Autodesk Inventor part; units mm, degrees
ref_plane "YZ Plane" through (0, 0, 0) normal (1, 0, 0) x (0, 1, 0)
ref_plane "XZ Plane" through (0, 0, 0) normal (0, 1, 0) x (-1, 0, 0)
ref_plane "XY Plane" through (0, 0, 0) normal (0, 0, 1) x (1, 0, 0)
sketch "Sketch1" plane through (0, 0, 0) normal (1, 0, 0) x (0, 1, 0)
  circle A0 centre (-31.75, 44.45) radius 11.1125
  circle A1 centre (-76.2, 44.45) radius 11.1125
  circle A2 centre (-101.6, 44.45) radius 11.1125
  line L0 (-130.175, 71.4375) -> (-92.075, 71.4375)
  arc A3 (-130.175, 71.4375) -> (-134.9375, 66.675) centre (-130.175, 66.675) ccw
  arc A4 (26.9875, 17.4625) -> (31.75, 22.225) centre (26.9875, 22.225) ccw
  line L1 (-130.175, 17.4625) -> (-92.075, 17.4625)
  circle A5 centre (25.4, 28.575) radius 2.1082
  circle A6 centre (-92.075, 66.675) radius 2.1082
  line L2 (31.75, 66.675) -> (31.75, 22.225)
  circle A7 centre (-92.075, 22.225) radius 2.1082
  arc A8 (-134.9375, 22.225) -> (-130.175, 17.4625) centre (-130.175, 22.225) ccw
  circle A9 centre (-130.175, 66.675) radius 2.1082
  line L3 (-134.9375, 66.675) -> (-134.9375, 22.225)
  circle A10 centre (-130.175, 22.225) radius 2.1082
  line L4 (-92.075, 71.4375) -> (26.9875, 71.4375)
  arc A11 (31.75, 66.675) -> (26.9875, 71.4375) centre (26.9875, 66.675) ccw
  circle A12 centre (26.9875, 66.675) radius 2.1345
  line L5 (-92.075, 17.4625) -> (26.9875, 17.4625)
  line L6 (26.9875, 66.675) -> (-17.4625, 66.675)
  line L7 (-17.4625, 66.675) -> (-11.1125, 66.675)
  line L8 (-17.4625, 66.675) -> (-23.8125, 66.675)
  circle A13 centre (-11.1125, 66.675) radius 2.1345
  line L9 (26.9875, 44.45) -> (6.6675, 44.45)
  circle A14 centre (6.6675, 44.45) radius 14.2875
  line L10 (-130.175, 22.225) -> (-92.075, 22.225)
  line L11 (-111.125, 22.225) -> (-111.125, 6.35)
  circle A15 centre (-111.125, 6.35) radius 2.1336
  line L12 (-111.125, 6.35) -> (-111.125, 0)
  line L13 (-111.125, 0) -> (-117.475, 0)
  line L14 (-111.125, 0) -> (-104.775, 0)
  line L15 (-117.475, 0) -> (-130.175, 17.4625)
  line L16 (-104.775, 0) -> (-92.075, 17.4625)
  line L17 (-130.175, 66.675) -> (-92.075, 66.675)
  line L18 (-111.125, 66.675) -> (-111.125, 82.55)
  circle A16 centre (-111.125, 82.55) radius 2.1336
  line L19 (-111.125, 82.55) -> (-111.125, 88.9)
  line L20 (-111.125, 88.9) -> (-117.475, 88.9)
  line L21 (-117.475, 88.9) -> (-104.775, 88.9)
  line L22 (-104.775, 88.9) -> (-92.075, 71.4375)
  line L23 (-117.475, 88.9) -> (-130.175, 71.4375)
  line L24 (26.9875, 71.4375) -> (55.5625, 71.4375)
  line L25 (55.5625, 71.4375) -> (55.5625, 58.7375)
  line L26 (55.5625, 58.7375) -> (31.75, 58.7375)
  line L27 (55.5625, 65.0875) -> (49.2125, 65.0875)
  circle A17 centre (49.2125, 65.0875) radius 2.1336
  point P0 (0, 0)
  point P1 (26.9875, 71.4375)
  dimension "d2" = 6.35
  dimension "d3" = 6.35
  dimension "d4" = 44.45
  dimension "d5" = 20.32
  dimension "d6" = 28.575
  dimension "d7" = 4.2672
  dimension "d8" = 6.35
  dimension "d9" = 6.35
  dimension "d10" = 6.35
  dimension "d11" = 15.875
  dimension "d12" = 4.2672
  dimension "d13" = 6.35
  dimension "d14" = 6.35
  dimension "d15" = 12.7
  dimension "d21" = 28.575
  dimension "d22" = 6.35
  dimension "d23" = 4.2672
extrude "Extrusion1" add sketch "Sketch1" along normal blind 3.175 contours L23 L20 L19 A16 L18 L0 | L0 L4 A11 L2 A4 L5 L1 A8 L3 A3 | L18 A16 L19 L21 L22 L0 | L24 L25 L26 L2 A11
fillet "Fillet1" radius 6.35 4 edges at (1.5875, -130.175, 71.4375) (1.5875, -117.475, 88.9) (1.5875, -104.775, 88.9) (1.5875, -92.075, 71.4375)
fillet "Fillet3" radius 6.35 3 edges at (1.5875, 31.75, 58.7375) (1.5875, 55.5625, 58.7375) (1.5875, 55.5625, 71.4375)
properties part number "winch plate"
Model file for the job. Use its own axes, mm. A direction names the side the tool comes from. Give positions to 0.01 mm unless a question says otherwise; leave off trailing zeros. Order: outer loops, then holes, each group sorted by start corner. A loop starts at its lowest first (then second) coordinate and runs counter-clockwise, first axis right, second up. Notation, with made-up numbers: (37.5, 86) -> (63.5, 86) arc R25 cw to (63.5, 118) -> close; hole circle Ø9 at (-13, -0.75). An arc over 180 degrees is marked (long way). Use CSV: the item, a comma, the result in double quotes.
1. Drop flat-ended pins along their axis: pin 1 (3.5 mm diameter, centred on y = -130.175, z = 66.675, fed in from -X) (3 decimals); pin 2 (1 mm diameter, centred on x = 2.5, z = 40, fed in from +Y). Give the stop position or say it passes through.
Outcome:
pin 1,"through"
pin 2,"y = 31.75"
2. 3-axis set-ups, long thin cutter, end or side, ignore diameter. For faces 4 (the cylindrical face through (1.565, -25.776, 35.08)), 5 (the flat face through (2, 31.75, 38)): which of +Z, -Z, +X, -X, +Y, -Y reach the whole face in a straight line?
Outcome:
face 4,"+X, -X"
face 5,"-Z, +X, -X, +Y"
3. Band-saw the part on B-B, the plane y = -76.2. Give the cut face in (x, z) (1 decimal).
Outcome:
outline,"(0, 17.5) -> (3.2, 17.5) -> (3.2, 33.3) -> (0, 33.3) -> close; (0, 55.6) -> (3.2, 55.6) -> (3.2, 71.4) -> (0, 71.4) -> close"
4. Mould opens along Y. For faces 1 (the flat face through (0, -41, 54)), 2 (the cylindrical face through (1.57, 30.39, 18.89)), 3 (the cylindrical face through (1.565, -128.164, 66.042)) say: +Y half, -Y half, draft (parallel to the pull), parting line (faces both ways), or undercut.
Outcome:
face 1,"draft"
face 2,"+Y half"
face 3,"undercut"
5. Drill centre lines: line 1 along Y through (x, z) = (1.6, 44); line 2 along Z through (x, y) = (0.6, -111.5); line 3 along Z through (x, y) = (0.8, -31.5). Where is each one in solid material? Low to high. Write a range as from..to.
Outcome:
line 1,"-134.94..-112.7, -90.5..-87.3, -65.1..-42.85, -20.65..-7.61, 20.95..31.75"
line 2,"17.46..39.4, 49.5..80.45, 84.65..88.9"
line 3,"17.46..33.34, 55.56..71.44"
6. Band-saw the part on A-A, the plane z = 44.45. Count the separate pieces of the cut face and the enclosed holes in it, then the cut area to 3 significant figures.
Outcome:
separate pieces,"5"
enclosed holes,"0"
area,"227 mm²"
7. Band-saw the part on D-D, the plane z = 82.55. Give the cut face in (x, y) (3 decimals), then the cut area to 3 significant figures.
Outcome:
outline,"(0, -122.093) -> (3.175, -122.093) -> (3.175, -113.259) -> (0, -113.259) -> close; (0, -108.991) -> (3.175, -108.991) -> (3.175, -100.157) -> (0, -100.157) -> close"
area,"56.1 mm²"
